Design review of the part built by this model. Coordinates are the model's own, in mm. A direction names the side the tool comes from. Round coordinates to 2 decimals unless told otherwise and drop trailing zeros. Order: outer loops, then holes, each group sorted by start corner. A loop starts at its lowest first (then second) coordinate and runs counter-clockwise, first axis right, second up. Notation, with made-up numbers: (70, 48.5) - (93, 48.5) arc R14 ccw to (93, 64.5) - close; hole circle Ø8 at (32.5, -17.75). An arc over 180 degrees is marked (long way). Use CSV: the item, a comma, the result in double quotes. Start each with the question number.
from build123d import *

# Parameters (mm, degrees)
SKETCH2_W           = 18
SKETCH2_H           = 18
SKETCH2_W_2         = 11
SKETCH2_H_2         = 11
SKETCH3_W           = 30
SKETCH3_H           = 30
SKETCH3_W_2         = 33.981635874
SKETCH3_H_2         = 34.73651567
BOSS_EXTRUDE1_DEPTH = 5
SKETCH4_W           = 50
SKETCH4_H           = 18
CUT_EXTRUDE1_DEPTH  = 4
SKETCH5_W           = 61.801380332
SKETCH5_H           = 123.620772257
CUT_EXTRUDE2_DEPTH  = 175
SKETCH6_W           = 30
SKETCH6_H           = 6
CUT_EXTRUDE3_DEPTH  = 10


with BuildPart() as part:
    # Sweep2: sweep along a path in Sketch1
    with BuildLine(Plane.XY) as sweep2_path:
        Line((0, 0), (0, 100))
        Line((0, 100), (320, 100))
        Line((320, 100), (320, 0))
    # Sketch2 → Sweep2 (sweep)
    with BuildSketch(Plane(origin=(0, 0, 0), x_dir=(1, 0, 0), z_dir=(0, 1, 0))):
        Rectangle(SKETCH2_W, SKETCH2_H)
        Rectangle(SKETCH2_W_2, SKETCH2_H_2, mode=Mode.SUBTRACT)
    sweep(path=sweep2_path.line, transition=Transition.RIGHT)

    # Sketch3 → Boss-Extrude1 (add)
    with BuildSketch(Plane(origin=(0, 0, 0), x_dir=(1, 0, 0), z_dir=(0, 1, 0))):
        Rectangle(SKETCH3_W, SKETCH3_H)
        with Locations((320, 0)):
            Rectangle(SKETCH3_W_2, SKETCH3_H_2)
    extrude(amount=-BOSS_EXTRUDE1_DEPTH)

    # Sketch4 → Cut-Extrude1 (cut)
    with BuildSketch(Plane.XZ.offset(-91)):
        with Locations((160, 0)):
            Rectangle(SKETCH4_W, SKETCH4_H)
    extrude(amount=-CUT_EXTRUDE1_DEPTH, mode=Mode.SUBTRACT)

    # Sketch5 → Cut-Extrude2 (cut)
    with BuildSketch(Plane(origin=(336.990817937, 0, 0), x_dir=(0, 0, -1), z_dir=(1, 0, 0))):
        with Locations((13.532432331, 56.810386129)):
            Rectangle(SKETCH5_W, SKETCH5_H)
    extrude(amount=-CUT_EXTRUDE2_DEPTH, mode=Mode.SUBTRACT)

    # Sketch6 → Cut-Extrude3 (cut)
    with BuildSketch(Plane(origin=(0, 0, 0), x_dir=(1, 0, 0), z_dir=(0, 1, 0))):
        with Locations((0, 12)):
            Rectangle(SKETCH6_W, SKETCH6_H)
    extrude(amount=-CUT_EXTRUDE3_DEPTH, mode=Mode.SUBTRACT)


solid = part.part
Q1. Take a section at A-A (y = 35.5). State the section outline as (x, z) points, plus the area to 3 significant figures.
Q2. Tool access review of faces 1 (the flat face through (-9, 55, 0)), 2 (the flat face through (51, 95, 9)), 3 (the flat face through (41, 96, -5.5)), 4 (the flat face through (9, 46, 0)): name each direction out of +Z, -Z, +X, -X, +Y, -Y from which nothing blocks a thin tool from reaching the whole face with its end or side.
Q3. Take a section at C-C (z = 2.5). State the section outline as (x, y) points, plus the area to 3 significant figures.
Q4. Take a section at D-D (y = 102.5). State the section outline as (x, z) points, plus the area to 3 significant figures.
Q5. Clearance check with flat-ended pins moving along their axes: pin 1 (1.5 mm diameter, centred on y = -3, z = -0.5, fed in from +X); pin 2 (8 mm diameter, centred on x = 5, y = 94.5, fed in from +Z); pin 3 (9 mm diameter, centred on y = 56, z = -1, fed in from +X). State where each tip first meets the part, or that it passes through.
Q6. The part is to be moulded in two halves that separate along X. For faces 5 (the flat face through (148, 95, -7)), 6 (the flat face through (-5.5, 53, 0)), 7 (the flat face through (0, 0, 0)), 8 (the flat face through (15, -2, 3)), say which applies: +X half, -X half, draft (parallel to the pull), parting line (faces both ways), or undercut.
Q7. Take a section at B-B (x = 145). State the section outline as (y, z) points.
Q8. For L1, parallel to Z at x = -0.5, y = 71; L2, parallel to X at y = 9, z = 8.5; L3, parallel to Y at x = 65, z = -0.5, list the stretches that pass through material, from the lowest coordinate up. Write a range as [from, to].
Findings below:
1,outline,"(-9, -9) - (9, -9) - (9, 9) - (-9, 9) - close; hole (-5.5, -5.5) - (5.5, -5.5) - (5.5, 5.5) - (-5.5, 5.5) - close"
1,area,"203 mm^2"
2,face 1,"+Z, -Z, -X, +Y"
2,face 2,"+Z, +X, -X, +Y"
2,face 3,"none"
2,face 4,"+Z, -Z, +X"
3,outline,"(-15, -5) - (15, -5) - (15, 0) - (9, 0) - (9, 91) - (135, 91) - (135, 94.5) - (5.5, 94.5) - (5.5, 0) - (-5.5, 0) - (-5.5, 105.5) - (161.99, 105.5) - (161.99, 109) - (-9, 109) - (-9, 0) - (-15, 0) - close"
3,area,"1,890 mm^2"
4,outline,"(-9, -9) - (161.99, -9) - (161.99, -5.5) - (-5.5, -5.5) - (-5.5, 5.5) - (161.99, 5.5) - (161.99, 9) - (-9, 9) - close"
4,area,"1,240 mm^2"
5,pin 1,"stops at x = 15"
5,pin 2,"stops at z = 9"
5,pin 3,"stops at x = 9"
6,face 5,"draft"
6,face 6,"undercut"
6,face 7,"undercut"
6,face 8,"+X half"
7,outline,"(95, -9) - (109, -9) - (109, 9) - (95, 9) - (95, 5.5) - (105.5, 5.5) - (105.5, -5.5) - (95, -5.5) - close"
8,L1,"z = [-9, -5.5], [5.5, 9]"
8,L2,"x = [-9, 9]"
8,L3,"y = [91, 94.5], [105.5, 109]"
